from build123d import *

# Parameters (mm, degrees)
SKETCH1_W           = 60
SKETCH1_H           = 43
SKETCH1_R           = 3
BOSS_EXTRUDE1_DEPTH = 8
FILLET1_R           = 4
SKETCH2_R           = 17
CUT_EXTRUDE1_DEPTH  = 1.6


with BuildPart() as part:
    # Sketch1 → Boss-Extrude1 (new body)
    with BuildSketch(Plane.XY):
        Rectangle(SKETCH1_W, SKETCH1_H)
        with Locations((23, 16)):
            Circle(SKETCH1_R, mode=Mode.SUBTRACT)
        with Locations(Location((23, -16, 0), (0, 0, 180))):
            Circle(SKETCH1_R, mode=Mode.SUBTRACT)
        with Locations((-23, -16)):
            Circle(SKETCH1_R, mode=Mode.SUBTRACT)
        with Locations(Location((-23, 16, 0), (0, 0, 180))):
            Circle(SKETCH1_R, mode=Mode.SUBTRACT)
    extrude(amount=BOSS_EXTRUDE1_DEPTH)

    # Fillet1
    fillet1_edges = [part.edges().sort_by_distance(p)[0] for p in [
        (30, -21.5, 4),
        (-30, -21.5, 4),
        (-30, 21.5, 4),
        (30, 21.5, 4),
    ]]
    fillet(fillet1_edges, radius=FILLET1_R)

    # Sketch2 → Cut-Extrude1 (cut)
    with BuildSketch(Plane.XY.offset(8)):
        Circle(SKETCH2_R)
    extrude(amount=-CUT_EXTRUDE1_DEPTH, mode=Mode.SUBTRACT)


solid = part.part
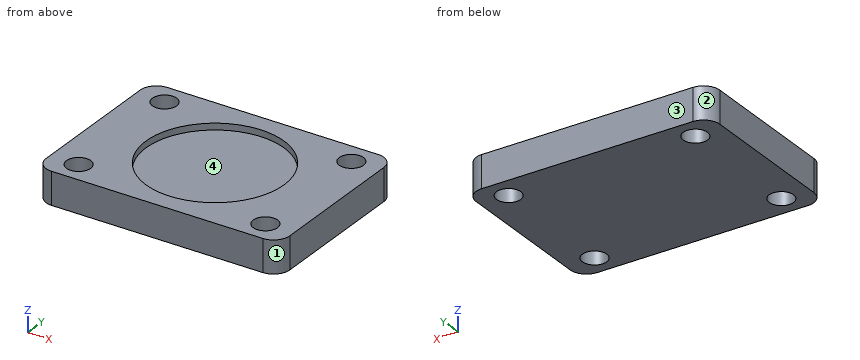
The model under review builds one solid part; all positions refer to its coordinate system, in mm. Face numbers are marked on the shaded views. Round coordinates to 2 decimals unless told otherwise and drop trailing zeros. Loops run counter-clockwise (first coordinate to the right, second up) from the corner with the lowest first, then second, coordinate; pieces in that order, holes last. Notation, with made-up numbers: M 16,37 L 31,37 A16 ccw 31,44 Z; hole C 63,38 d10. An arc over 180 degrees is marked long. Answer as a JSON object with one key per item and string values.
Item 1: Clearance check with a flat-ended pin moving along its axis: P1, Ø10, axis at x = 8, y = -2, coming from the +Z side. State where the tip first meets the part, or that it passes through.
Check sheet entries:
{"P1": "z = 6.4"}
Item 2: For line 1 along Y through (x, z) = (-23, 5.75); line 2 along Y through (x, z) = (25.5, 3); line 3 along Y through (x, z) = (0, 7.6), list the stretches that pass through material, from the lowest coordinate up.
Check sheet entries:
{"line 1": "-21.5 to -19, -13 to 13, 19 to 21.5", "line 2": "-21.5 to -17.66, -14.34 to 14.34, 17.66 to 21.5", "line 3": "-21.5 to -17, 17 to 21.5"}
Item 3: We need section B-B, the plane z = 2. State the section outline as (x, y) points, and give its area (3 significant figures).
Check sheet entries:
{"outline": "M -30,-17.5 A4 ccw -26,-21.5 L 26,-21.5 A4 ccw 30,-17.5 L 30,17.5 A4 ccw 26,21.5 L -26,21.5 A4 ccw -30,17.5 Z; hole C -23,-16 d6; hole C -23,16 d6; hole C 23,-16 d6; hole C 23,16 d6", "area": "2,450 mm2"}
Item 4: We need section A-A, the plane x = -23. State the section outline as (y, z) points, and give its area (3 significant figures).
Check sheet entries:
{"outline": "M -21.5,0 L -19,0 L -19,8 L -21.5,8 Z; M -13,0 L 13,0 L 13,8 L -13,8 Z; M 19,0 L 21.5,0 L 21.5,8 L 19,8 Z", "area": "248 mm2"}
Item 5: The part is to be moulded in two halves that separate along X. For the marked faces 1, 2, 3 and 4, say which applies: +X half, -X half, draft (parallel to the pull), parting line (faces both ways), or undercut.
Check sheet entries:
{"face 1": "+X half", "face 2": "-X half", "face 3": "draft", "face 4": "undercut"}
Item 6: We need section C-C, the plane z = 7. State the section outline as (x, y) points.
Check sheet entries:
{"outline": "M -30,-17.5 A4 ccw -26,-21.5 L 26,-21.5 A4 ccw 30,-17.5 L 30,17.5 A4 ccw 26,21.5 L -26,21.5 A4 ccw -30,17.5 Z; hole C -23,-16 d6; hole C -23,16 d6; hole C 0,0 d34; hole C 23,-16 d6; hole C 23,16 d6"}
Item 7: We need section D-D, the plane y = 16. State the section outline as (x, z) points, and give its area (3 significant figures).
Check sheet entries:
{"outline": "M -30,0 L -26,0 L -26,8 L -30,8 Z; M -20,0 L 20,0 L 20,8 L 5.74,8 L 5.74,6.4 L -5.74,6.4 L -5.74,8 L -20,8 Z; M 26,0 L 30,0 L 30,8 L 26,8 Z", "area": "366 mm2"}
